Verification items for this drawing (mm, ordinates from the low corner). Round coordinates to 2 decimals unless told otherwise and drop trailing zeros. Write each loop counter-clockwise with the first axis right and the second up, starting at its lowest first coordinate (ties: lowest second). Pieces come first, ordered by that corner, then holes.
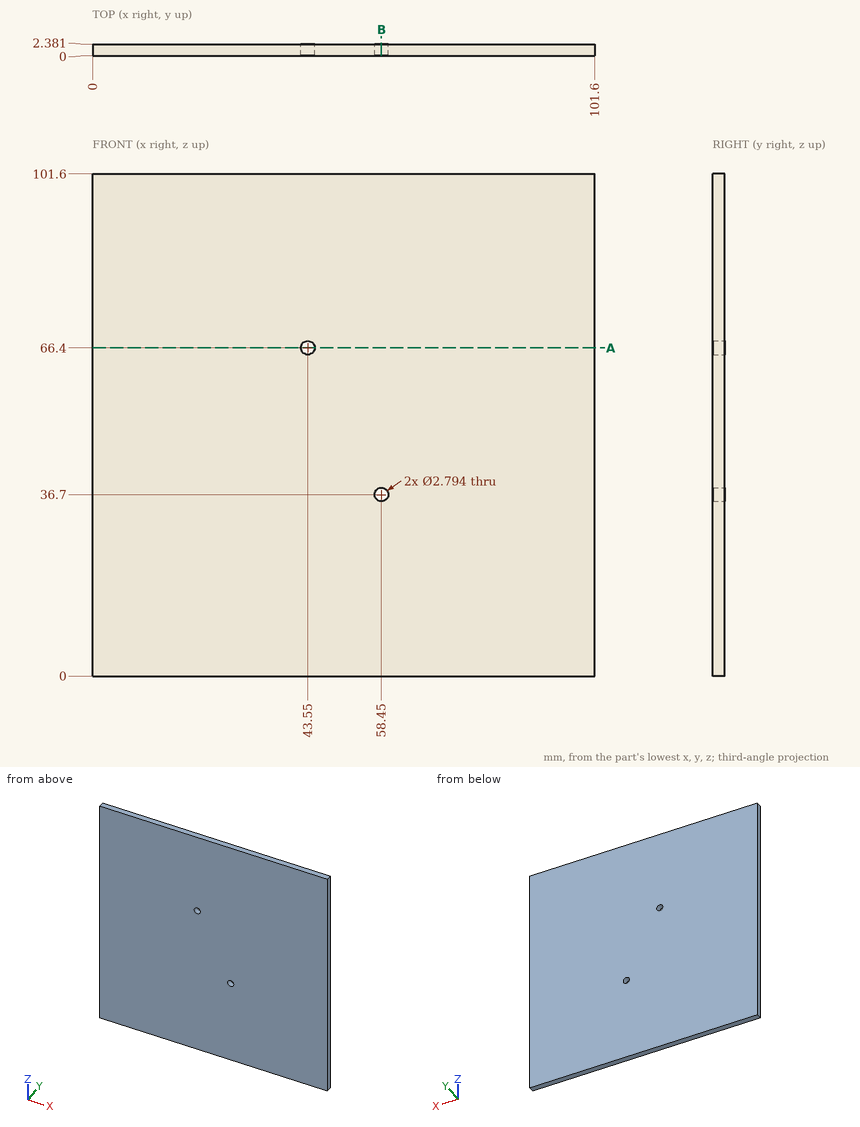
1. Depth check by flat-ended pin: pin 1 Ø2 at (x, z) = (58.45, 36.7) entering from +Y. Enter the tip coordinate at first touch or a pass-through.
2. Scan lines: line 1 along Z through (x, y) = (43.55, 1.7); line 2 along Z through (x, y) = (58.45, 1.65); line 3 along X through (y, z) = (1.65, 36.7). Record each from-to range of solid material in increasing order.
3. Section check A-A (z = 66.4). Record the cut outline in (x, y).
4. Section check B-B (x = 58.45). Record the cut outline in (y, z).
Results below:
1. pin 1: passes through
2. line 1: z = 0 to 65, 67.8 to 101.6
2. line 2: z = 0 to 35.3, 38.1 to 101.6
2. line 3: x = 0 to 57.05, 59.85 to 101.6
3. outline: (0, 0) - (42.15, 0) - (42.15, 2.38) - (0, 2.38) - close; (44.95, 0) - (101.6, 0) - (101.6, 2.38) - (44.95, 2.38) - close
4. outline: (0, 0) - (2.38, 0) - (2.38, 35.3) - (0, 35.3) - close; (0, 38.1) - (2.38, 38.1) - (2.38, 101.6) - (0, 101.6) - close
